```python
from build123d import *

# Parameters (mm, degrees)
SKETCH1_W           = 127
SKETCH1_H           = 127
BOSS_EXTRUDE1_DEPTH = 2.9972
SKETCH2_W           = 63.5
SKETCH2_H           = 2.9972
SKETCH2_W_2         = 2.9972
SKETCH2_H_2         = 63.5
CUT_EXTRUDE1_DEPTH  = 2.9972
CUT_EXTRUDE2_REACH  = 181.63


with BuildPart() as part:
    # Sketch1 → Boss-Extrude1 (new body)
    with BuildSketch(Plane(origin=(0, 0, 0), x_dir=(1, 0, 0), z_dir=(0, 1, 0))):
        with Locations((63.5, -63.5)):
            Rectangle(SKETCH1_W, SKETCH1_H)
    extrude(amount=BOSS_EXTRUDE1_DEPTH)

    # Sketch2 → Cut-Extrude1 (cut)
    with BuildSketch(Plane(origin=(0, 2.9972, 0), x_dir=(1, 0, 0), z_dir=(0, 1, 0))):
        with Locations((63.5, -125.5014)):
            Rectangle(SKETCH2_W, SKETCH2_H)
        with Locations((1.4986, -63.5)):
            Rectangle(SKETCH2_W_2, SKETCH2_H_2)
        with Locations((125.5014, -63.5)):
            Rectangle(SKETCH2_W_2, SKETCH2_H_2)
        with Locations((63.5, -1.4986)):
            Rectangle(SKETCH2_W, SKETCH2_H)
    extrude(amount=-CUT_EXTRUDE1_DEPTH, mode=Mode.SUBTRACT)

    # Sketch3 → Cut-Extrude2 (cut, up to next)
    with BuildSketch(Plane(origin=(0, 2.9972, 0), x_dir=(1, 0, 0), z_dir=(0, 1, 0)), mode=Mode.PRIVATE) as cut_extrude2_sk1:
        Polygon((2.9972, -64.897), (8.2042, -64.897), (8.2042, -66.675), (10.4902, -66.675), (10.4902, -64.897), (15.6972, -64.897), (15.6972, -62.103), (10.4902, -62.103), (10.4902, -60.325), (8.2042, -60.325), (8.2042, -62.103), (2.9972, -62.103), align=None)
    cut_extrude2_tool1 = extrude(cut_extrude2_sk1.sketch, amount=-CUT_EXTRUDE2_REACH, mode=Mode.PRIVATE) & part.part
    # Sketch3 → Cut-Extrude2 (cut, up to next)
    with BuildSketch(Plane(origin=(0, 2.9972, 0), x_dir=(1, 0, 0), z_dir=(0, 1, 0)), mode=Mode.PRIVATE) as cut_extrude2_sk2:
        Polygon((62.103, -124.0028), (64.897, -124.0028), (64.897, -118.7958), (66.675, -118.7958), (66.675, -116.5098), (64.897, -116.5098), (64.897, -111.3028), (62.103, -111.3028), (62.103, -116.5098), (60.325, -116.5098), (60.325, -118.7958), (62.103, -118.7958), align=None)
    cut_extrude2_tool2 = extrude(cut_extrude2_sk2.sketch, amount=-CUT_EXTRUDE2_REACH, mode=Mode.PRIVATE) & part.part
    # Sketch3 → Cut-Extrude2 (cut, up to next)
    with BuildSketch(Plane(origin=(0, 2.9972, 0), x_dir=(1, 0, 0), z_dir=(0, 1, 0)), mode=Mode.PRIVATE) as cut_extrude2_sk3:
        Polygon((118.7958, -66.675), (118.7958, -64.897), (124.0028, -64.897), (124.0028, -62.103), (118.7958, -62.103), (118.7958, -60.325), (116.5098, -60.325), (116.5098, -62.103), (111.3028, -62.103), (111.3028, -64.897), (116.5098, -64.897), (116.5098, -66.675), align=None)
    cut_extrude2_tool3 = extrude(cut_extrude2_sk3.sketch, amount=-CUT_EXTRUDE2_REACH, mode=Mode.PRIVATE) & part.part
    # Sketch3 → Cut-Extrude2 (cut, up to next)
    with BuildSketch(Plane(origin=(0, 2.9972, 0), x_dir=(1, 0, 0), z_dir=(0, 1, 0)), mode=Mode.PRIVATE) as cut_extrude2_sk4:
        Polygon((62.103, -2.9972), (62.103, -8.2042), (60.325, -8.2042), (60.325, -10.4902), (62.103, -10.4902), (62.103, -15.6972), (64.897, -15.6972), (64.897, -10.4902), (66.675, -10.4902), (66.675, -8.2042), (64.897, -8.2042), (64.897, -2.9972), align=None)
    cut_extrude2_tool4 = extrude(cut_extrude2_sk4.sketch, amount=-CUT_EXTRUDE2_REACH, mode=Mode.PRIVATE) & part.part
    add(cut_extrude2_tool1.solids().sort_by_distance((9.3472, 2.9972, 63.5))[0], mode=Mode.SUBTRACT)
    add(cut_extrude2_tool2.solids().sort_by_distance((63.5, 2.9972, 117.6528))[0], mode=Mode.SUBTRACT)
    add(cut_extrude2_tool3.solids().sort_by_distance((117.6528, 2.9972, 63.5))[0], mode=Mode.SUBTRACT)
    add(cut_extrude2_tool4.solids().sort_by_distance((63.5, 2.9972, 9.3472))[0], mode=Mode.SUBTRACT)


solid = part.part
```
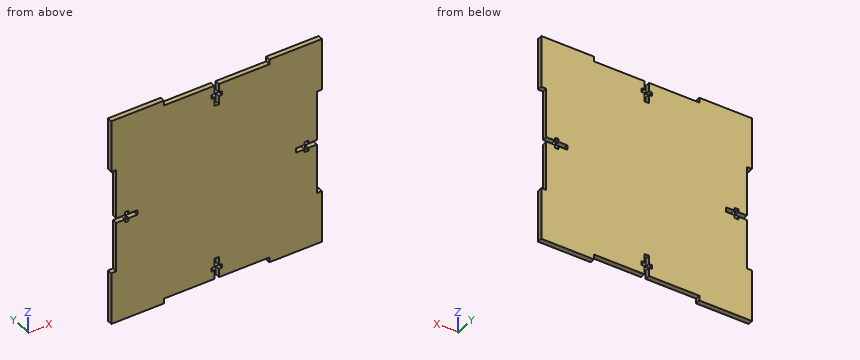
Geometry check sheet. Reference: the model listing, model coordinates, mm. Coordinates: 2 decimals unless noted, no trailing zeros. Write each loop counter-clockwise with the first axis right and the second up, starting at its lowest first coordinate (ties: lowest second). Pieces come first, ordered by that corner, then holes. Notation, with made-up numbers: M 77,-11 L 90,-11 A14 cw 90,2 Z; hole C -32.75,48 d2. An arc over 180 degrees is marked long. Use one line per item in the form item = value. Start each with the question number.
1) Section check A-A on z = 83.5. Enter the section's corners in (x, y), and give its area (3 significant figures).
2) Section check B-B on x = 55. Enter the section's corners in (y, z), and give its area (3 significant figures).
3) Thickness scan on probe 1 along X at (y, z) = (2.7, 12.5); probe 2 along X at (y, z) = (2.4, 72); probe 3 along Z at (x, y) = (62.5, 2.05). Record the ranges inside material, lowest first. Write a range as from..to.
4) Go/stop test with flat-tipped pins: pin 1 Ø1 at (x, y) = (84.5, 0.5) entering from +Z; pin 2 Ø1.4 at (x, y) = (63, 2) entering from -Z; pin 3 Ø1.4 at (y, z) = (2, 63.5) entering from -X. Record where each tip stops, or that it passes through.
Responses:
q1.outline = M 3,0 L 124,0 L 124,3 L 3,3 Z
q1.area = 363 mm2
q2.outline = M 0,3 L 3,3 L 3,124 L 0,124 Z
q2.area = 363 mm2
q3.probe_1 = 0..62.1, 64.9..127
q3.probe_2 = 3..124
q3.probe_3 = 15.7..111.3
q4.pin_1 = 124
q4.pin_2 = 15.7
q4.pin_3 = 15.7
